Geometry check sheet. Reference: the model listing, model coordinates, mm. Face numbers are marked on the shaded views. A direction names the side the tool comes from. Round coordinates to 2 decimals unless told otherwise and drop trailing zeros. Loops run counter-clockwise (first coordinate to the right, second up) from the corner with the lowest first, then second, coordinate; pieces in that order, holes last.
```python
from build123d import *

# Parameters (mm, degrees)
SKETCH046_R     = 2.5
PAD023_DEPTH    = 2.5
SKETCH047_R     = 5
PAD024_DEPTH    = 3
FILLET003_R     = 1.5
SKETCH049_R     = 2.5
PAD025_DEPTH    = 4
SKETCH050_R     = 1.5
POCKET026_DEPTH = 4
PAD059_DEPTH    = 0.2


with BuildPart() as part:
    # Sketch046 → Pad023 (new body)
    with BuildSketch(Plane(origin=(0, 0, 30), x_dir=(1, 0, 0), z_dir=(0, 0, -1))):
        with Locations((101, 55)):
            Circle(SKETCH046_R)
    extrude(amount=-PAD023_DEPTH)

    # Sketch047 (on Face3 of Pad023) → Pad024 (join)
    with BuildSketch(Plane.XY.offset(32.5)):
        with Locations((101, -55)):
            Circle(SKETCH047_R)
    extrude(amount=PAD024_DEPTH)

    # Fillet003
    fillet003_edges = [part.edges().sort_by_distance(p)[0] for p in [
        (96, -55, 35.5),
    ]]
    fillet(fillet003_edges, radius=FILLET003_R)

    # Sketch049 → Pad025 (join)
    with BuildSketch(Plane(origin=(0, 0, 30), x_dir=(1, 0, 0), z_dir=(0, 0, -1))):
        with Locations((101, 55)):
            Circle(SKETCH049_R)
    extrude(amount=PAD025_DEPTH)

    # Sketch050 (on Face17 of Pad025) → Pocket026 (cut)
    with BuildSketch(Plane(origin=(0, 0, 26), x_dir=(1, 0, 0), z_dir=(0, 0, -1))):
        with Locations((101, 55)):
            Circle(SKETCH050_R)
    extrude(amount=-POCKET026_DEPTH, mode=Mode.SUBTRACT)


with BuildPart() as part_1:
    # Body002 placement: moved
    add(part.part.moved(Location((75, 0, 0))))

    # Sketch093 (on Face4 of Clone007) → Pad059 (new body)
    with BuildSketch(Plane(origin=(75, 0, 35.5), x_dir=(1, 0, 0), z_dir=(0, 0, 1))):
        Polygon((99.5, -53), (99, -53.5), (100.5, -55), (99, -56.5), (99.5, -57), (101, -55.5), (102.5, -57), (103, -56.5), (101.5, -55), (103, -53.5), (102.5, -53), (101, -54.5), align=None)
    extrude(amount=PAD059_DEPTH)


with BuildPart() as part_2:
    # Body016 placement: moved
    add(part_1.part.moved(Location((-52.5, 22, 0))))


solid = part_2.part
```
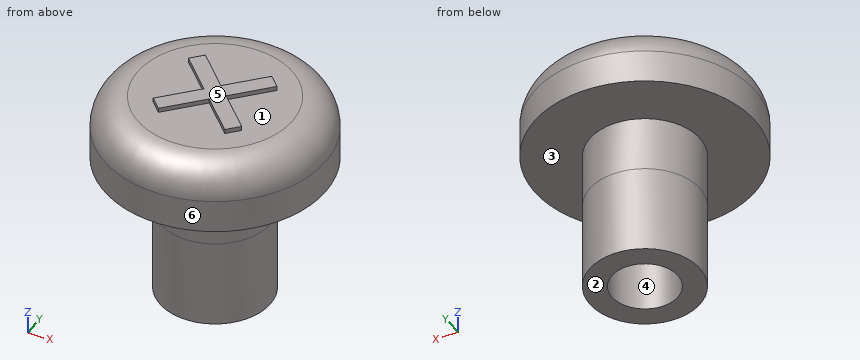
1) Sectioned sample at B-B, the plane z = 28.5. Record the cut outline in (x, y).
Report:
outline: circle Ø5 at (123.5, -33); hole circle Ø3 at (123.5, -33)
2) Scan lines: line 1 along X through (y, z) = (-33, 27.6); line 2 along Y through (x, z) = (123.5, 27.9); line 3 along Z through (x, y) = (125, -33.5). Record each from-to range of solid material in increasing order.
Report:
line 1: x = 121 to 122, 125 to 126
line 2: y = -35.5 to -34.5, -31.5 to -30.5
line 3: z = 26 to 35.5
3) Access from +Z, -Z, +X, -X, +Y, -Y to the whole of each face (thin tool, end or side, straight path). Record for the marked faces 1, 2 and 3.
Report:
face 1: +Z
face 2: -Z, +X, -X, +Y, -Y
face 3: -Z
4) Sectioned sample at C-C, the plane z = 35. Record the cut outline in (x, y), then the cut area to 3 significant figures.
Report:
outline: circle Ø9.24 at (123.5, -33)
area: 67.0 mm2
5) Mould release check, pull along X, two halves, no side actions. Record for the marked faces 4, 5 and 6: +X half, -X half, draft (parallel to the pull), parting line (faces both ways), or undercut.
Report:
face 4: undercut
face 5: draft
face 6: parting line
6) Gauge pin test, flat ends, axial feed: pin 1 (1.5 mm diameter, centred on x = 126, z = 29.5, fed in from -Y); pin 2 (2.5 mm diameter, centred on x = 123.5, y = -33, fed in from -Z); pin 3 (1.5 mm diameter, centred on x = 126, z = 30.5, fed in from +Y). Record the tip position at first contact, or that the pin passes through.
Report:
pin 1: stops at y = -34.79
pin 2: stops at z = 30
pin 3: stops at y = -31.21
7) Sectioned sample at A-A, the plane z = 31. Record the cut outline in (x, y), then the cut area to 3 significant figures.
Report:
outline: circle Ø5 at (123.5, -33)
area: 19.6 mm2
